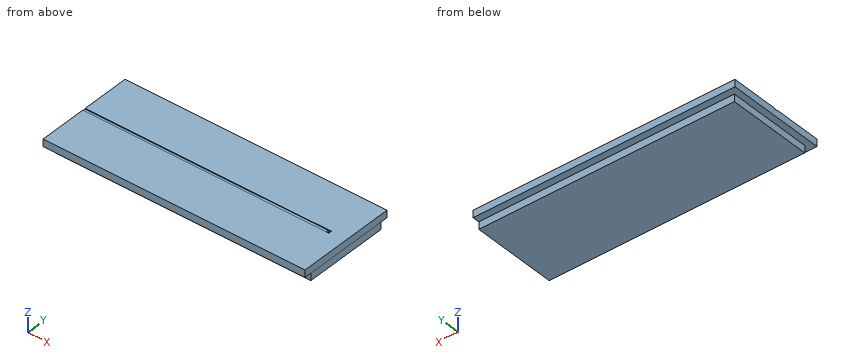
```python
from build123d import *

# Parameters (mm, degrees)
F6_W     = 56.56732
F6_H     = 21.370728
F6_R     = 0.301175
F7_DEPTH = 0.3048
F8_DEPTH = 0.1524
F5_W     = 56.56732
F5_H     = 21.370728
F9_DEPTH = 1.0922
F3_W     = 55.18673
F3_H     = 18.370153
F4_DEPTH = 1.5494


with BuildPart() as f7:
    # F6 (on face) → F7 (new body)
    with BuildSketch(Plane.XY):
        Rectangle(F6_W, F6_H)
        with Locations((24.477545, 0)):
            Circle(F6_R, mode=Mode.SUBTRACT)
    extrude(amount=F7_DEPTH)

    # F1 (on face) → F8 (join)
    with BuildSketch(Plane.XY.offset(0.3048)):
        Polygon((-24.833549, -0.31923), (-24.833549, -0.319519), (-28.28366, -0.319519), (-28.28366, -10.685364), (28.28366, -10.685364), (28.28366, 10.685364), (-28.28366, 10.685364), (-28.28366, 0.318926), (-24.833655, 0.318926), (-24.833655, 0.31923), (24.833655, 0.31923), (24.833655, -0.31923), align=None)
    extrude(amount=F8_DEPTH)

    # F5 (on Top) → F9 (join)
    with BuildSketch(Plane.XY):
        Rectangle(F5_W, F5_H)
    extrude(amount=-F9_DEPTH)

    # F3 (on face) → F4 (join)
    with BuildSketch(Plane(origin=(0, 0, -1.0922), x_dir=(1, 0, 0), z_dir=(0, 0, -1))):
        with Locations((0.690263, 0.001336)):
            Rectangle(F3_W, F3_H)
    extrude(amount=F4_DEPTH)


solid = f7.part
```
Work out the finished part from the listing and answer in its coordinate system (mm). Give positions to 0.01 mm unless a question says otherwise; leave off trailing zeros. Order: outer loops, then holes, each group sorted by start corner. A loop starts at its lowest first (then second) coordinate and runs counter-clockwise, first axis right, second up.
1. This flat-tipped pin is pushed along its axis until it touches: P1, Ø1.2, axis at y = 2, z = -2, coming from the -X side. Where does it stop, or does it pass through?
Result sheet:
P1: stops at x = -26.9
2. Section B-B, the plane z = -1.6 is taken. Determine the outline of the cut face in (x, y).
Result sheet:
outline: (-26.9, -9.19) - (28.28, -9.19) - (28.28, 9.18) - (-26.9, 9.18) - close
3. Straight lines are drawn through the part: L1, parallel to Y at x = -23.5, z = -1.25; L2, parallel to X at y = -2.25, z = -1.45; L3, parallel to Z at x = 21, y = 0. For each, find the intervals that lie inside material, in ascending order.
Result sheet:
L1: y = -9.19 to 9.18
L2: x = -26.9 to 28.28
L3: z = -2.64 to 0.3
4. Section A-A, the plane x = -20.5 is taken. Determine the outline of the cut face in (y, z).
Result sheet:
outline: (-10.69, -1.09) - (-9.19, -1.09) - (-9.19, -2.64) - (9.18, -2.64) - (9.18, -1.09) - (10.69, -1.09) - (10.69, 0.46) - (0.32, 0.46) - (0.32, 0.3) - (-0.32, 0.3) - (-0.32, 0.46) - (-10.69, 0.46) - close
